Build history of the part. All positions in model axes, mm. A direction names the side the tool comes from. Give positions to 0.01 mm unless a question says otherwise; leave off trailing zeros. Order: outer loops, then holes, each group sorted by start corner. A loop starts at its lowest first (then second) coordinate and runs counter-clockwise, first axis right, second up. Notation, with made-up numbers: (29.5, 85) - (55.5, 85) arc R24 cw to (55.5, 107) - close; hole circle Ø4 at (-20, 47.5). An arc over 180 degrees is marked (long way). Answer in a Markdown table with one row per item.
```python
from build123d import *

# Parameters (mm, degrees)
EXTRUDE_1_DEPTH            = 25.5
CUT_EXTRUDE_1_DEPTH        = 23
CUT_EXTRUDE_START          = -1.5
CUT_EXTRUDE_2_DEPTH        = 1.5
SKETCH_3_W                 = 9
SKETCH_3_H                 = 1.25
EXTRUDE_2_DEPTH            = 7
SKETCH_4_W                 = 9
SKETCH_4_H                 = 3
EXTRUDE_3_DEPTH            = 1.25
CHAMFER_1_SIZE             = 1.3
CHAMFER_1_OF_MIRROR_1_SIZE = 1.3
MIRROR_START               = -31
MIRROR_4_DEPTH             = 9
MIRROR_START_2             = 22
MIRROR_4_2_DEPTH           = 9
SKETCH_5_W                 = 75
SKETCH_5_H                 = 50
CUT_EXTRUDE_3_DEPTH        = 0.5
CUT_EXTRUDE_4_DEPTH        = 115.248905903
CUT_EXTRUDE_4_DEPTH_BACK   = 0.5
SKETCH_6_W                 = 50
SKETCH_6_H                 = 14.5
CUT_EXTRUDE_5_REACH        = 98.222
SKETCH_7_R                 = 1.5
CUT_EXTRUDE_6_REACH        = 116.249
CUT_EXTRUDE_7_REACH        = 116.249


# Read off the part's stored shape, not the designer's step: Зеркальное отражение4
with BuildPart() as part:
    # Эскиз1 → Бобышка-Вытянуть1 (new body)
    with BuildSketch(Plane(origin=(0, 0, 0), x_dir=(1, 0, 0), z_dir=(0, 1, 0))):
        with BuildLine():
            Line((-43.5, 37.25), (43.5, 37.25))
            ThreePointArc((43.5, 37.25), (49.156854249, 34.906854249), (51.5, 29.25))
            Line((51.5, 29.25), (51.5, -29.25))
            ThreePointArc((51.5, -29.25), (49.156854249, -34.906854249), (43.5, -37.25))
            Line((43.5, -37.25), (-43.5, -37.25))
            ThreePointArc((-43.5, -37.25), (-49.156854249, -34.906854249), (-51.5, -29.25))
            Line((-51.5, -29.25), (-51.5, 29.25))
            ThreePointArc((-51.5, 29.25), (-49.156854249, 34.906854249), (-43.5, 37.25))
        make_face()
    extrude(amount=EXTRUDE_1_DEPTH)

    # Эскиз2 → Вырез-Вытянуть1 (cut)
    with BuildSketch(Plane(origin=(0, 25.5, 0), x_dir=(1, 0, 0), z_dir=(0, 1, 0))):
        with BuildLine():
            Line((-49, 29.25), (-49, -29.25))
            ThreePointArc((-49, -29.25), (-47.389087297, -33.139087297), (-43.5, -34.75))
            Line((-43.5, -34.75), (43.5, -34.75))
            ThreePointArc((43.5, -34.75), (47.389087297, -33.139087297), (49, -29.25))
            Line((49, -29.25), (49, 29.25))
            ThreePointArc((49, 29.25), (47.389087297, 33.139087297), (43.5, 34.75))
            Line((43.5, 34.75), (-43.5, 34.75))
            ThreePointArc((-43.5, 34.75), (-47.389087297, 33.139087297), (-49, 29.25))
        make_face()
    extrude(amount=-CUT_EXTRUDE_1_DEPTH, mode=Mode.SUBTRACT)

    # Эскиз2<3> → Вырез-Вытянуть2 (cut)
    with BuildSketch(Plane(origin=(0, 25.5, 0), x_dir=(1, 0, 0), z_dir=(0, 1, 0)).offset(CUT_EXTRUDE_START)):
        with BuildLine():
            Line((51.5, -29.25), (51.5, 29.25))
            ThreePointArc((51.5, 29.25), (49.156854249, 34.906854249), (43.5, 37.25))
            Line((43.5, 37.25), (-43.5, 37.25))
            ThreePointArc((-43.5, 37.25), (-49.156854249, 34.906854249), (-51.5, 29.25))
            Line((-51.5, 29.25), (-51.5, -29.25))
            ThreePointArc((-51.5, -29.25), (-49.156854249, -34.906854249), (-43.5, -37.25))
            Line((-43.5, -37.25), (43.5, -37.25))
            ThreePointArc((43.5, -37.25), (49.156854249, -34.906854249), (51.5, -29.25))
        make_face()
        with BuildLine():
            ThreePointArc((43.5, -36), (48.272970773, -34.022970773), (50.25, -29.25))
            Line((50.25, -29.25), (50.25, 29.25))
            ThreePointArc((50.25, 29.25), (48.272970773, 34.022970773), (43.5, 36))
            Line((43.5, 36), (-43.5, 36))
            ThreePointArc((-43.5, 36), (-48.272970773, 34.022970773), (-50.25, 29.25))
            Line((-50.25, 29.25), (-50.25, -29.25))
            ThreePointArc((-50.25, -29.25), (-48.272970773, -34.022970773), (-43.5, -36))
            Line((-43.5, -36), (43.5, -36))
        make_face(mode=Mode.SUBTRACT)
    extrude(amount=CUT_EXTRUDE_2_DEPTH, mode=Mode.SUBTRACT)

    # Эскиз3 → Бобышка-Вытянуть2 (add)
    with BuildSketch(Plane(origin=(0, 25.5, 0), x_dir=(1, 0, 0), z_dir=(0, 1, 0))):
        with Locations((-26.5, -35.375)):
            Rectangle(SKETCH_3_W, SKETCH_3_H)
    extrude_2 = extrude(amount=EXTRUDE_2_DEPTH)

    # Эскиз4 → Бобышка-Вытянуть3 (add, through all)
    with BuildSketch(Plane.XY.offset(36)):
        with Locations((-26.5, 31)):
            Rectangle(SKETCH_4_W, SKETCH_4_H)
    extrude_3 = extrude(amount=EXTRUDE_3_DEPTH)

    # Фаска1
    chamfer_1_edges = [part.edges().sort_by_distance(p)[0] for p in [
        (-26.5, 32.5, 37.25),
    ]]
    chamfer(chamfer_1_edges, length=CHAMFER_1_SIZE)

    # Зеркальное отражение1: Бобышка-Вытянуть2, Бобышка-Вытянуть3 across plane
    add(extrude_2.mirror(Plane(origin=(0, 0, 0), x_dir=(0, 0, 1), z_dir=(1, 0, 0))))
    add(extrude_3.mirror(Plane(origin=(0, 0, 0), x_dir=(0, 0, 1), z_dir=(1, 0, 0))))

    # Фаска1 of Зеркальное отражение1
    chamfer_1_of_mirror_1_edges = [part.edges().sort_by_distance(p)[0] for p in [
        (26.5, 32.5, 37.25),
    ]]
    chamfer(chamfer_1_of_mirror_1_edges, length=CHAMFER_1_OF_MIRROR_1_SIZE)

    # Зеркальное отражение4 outline → Зеркальное отражение4 (add)
    with BuildSketch(Plane.YZ.offset(MIRROR_START)):
        Polygon((25.5, -34.75), (25.5, -36), (29.5, -36), (29.5, -37.25), (31.2, -37.25), (32.5, -35.95), (32.5, -34.75), align=None)
    extrude(amount=MIRROR_4_DEPTH)

    # Mirror 4 2 outline → Mirror 4 2 (add)
    with BuildSketch(Plane.YZ.offset(MIRROR_START_2)):
        Polygon((25.5, -34.75), (25.5, -36), (29.5, -36), (29.5, -37.25), (31.2, -37.25), (32.5, -35.95), (32.5, -34.75), align=None)
    extrude(amount=MIRROR_4_2_DEPTH)

    # Эскиз5 → Вырез-Вытянуть3 (cut)
    with BuildSketch(Plane.XZ):
        Rectangle(SKETCH_5_W, SKETCH_5_H)
    extrude(amount=-CUT_EXTRUDE_3_DEPTH, mode=Mode.SUBTRACT)

    # Эскиз6 → Вырез-Вытянуть4 (cut, two sides: drawn at the far end of the back side and taken through both)
    with BuildSketch(Plane(origin=(51.5, 0, 0), x_dir=(0, 0, -1), z_dir=(1, 0, 0)).offset(-CUT_EXTRUDE_4_DEPTH_BACK)):
        with Locations((0, 16.75)):
            Rectangle(SKETCH_6_W, SKETCH_6_H)
    extrude(amount=CUT_EXTRUDE_4_DEPTH + CUT_EXTRUDE_4_DEPTH_BACK, mode=Mode.SUBTRACT)

    # Эскиз7 → Вырез-Вытянуть5 (cut, up to next)
    with BuildSketch(Plane(origin=(0, 0, -37.25), x_dir=(-1, 0, 0), z_dir=(0, 0, -1)), mode=Mode.PRIVATE) as cut_extrude_5_sk1:
        with Locations((15.3, 21.7)):
            Circle(SKETCH_7_R)
    cut_extrude_5_tool1 = extrude(cut_extrude_5_sk1.sketch, amount=-CUT_EXTRUDE_5_REACH, mode=Mode.PRIVATE) & part.part
    # Эскиз7 → Вырез-Вытянуть5 (cut, up to next)
    with BuildSketch(Plane(origin=(0, 0, -37.25), x_dir=(-1, 0, 0), z_dir=(0, 0, -1)), mode=Mode.PRIVATE) as cut_extrude_5_sk2:
        with Locations((7.3, 21.7)):
            Circle(SKETCH_7_R)
    cut_extrude_5_tool2 = extrude(cut_extrude_5_sk2.sketch, amount=-CUT_EXTRUDE_5_REACH, mode=Mode.PRIVATE) & part.part
    # Эскиз7 → Вырез-Вытянуть5 (cut, up to next)
    with BuildSketch(Plane(origin=(0, 0, -37.25), x_dir=(-1, 0, 0), z_dir=(0, 0, -1)), mode=Mode.PRIVATE) as cut_extrude_5_sk3:
        with Locations((-0.7, 21.7)):
            Circle(SKETCH_7_R)
    cut_extrude_5_tool3 = extrude(cut_extrude_5_sk3.sketch, amount=-CUT_EXTRUDE_5_REACH, mode=Mode.PRIVATE) & part.part
    # Эскиз7 → Вырез-Вытянуть5 (cut, up to next)
    with BuildSketch(Plane(origin=(0, 0, -37.25), x_dir=(-1, 0, 0), z_dir=(0, 0, -1)), mode=Mode.PRIVATE) as cut_extrude_5_sk4:
        with Locations((-8.7, 21.7)):
            Circle(SKETCH_7_R)
    cut_extrude_5_tool4 = extrude(cut_extrude_5_sk4.sketch, amount=-CUT_EXTRUDE_5_REACH, mode=Mode.PRIVATE) & part.part
    add(cut_extrude_5_tool1.solids().sort_by_distance((-15.3, 21.7, -37.25))[0], mode=Mode.SUBTRACT)
    add(cut_extrude_5_tool2.solids().sort_by_distance((-7.3, 21.7, -37.25))[0], mode=Mode.SUBTRACT)
    add(cut_extrude_5_tool3.solids().sort_by_distance((0.7, 21.7, -37.25))[0], mode=Mode.SUBTRACT)
    add(cut_extrude_5_tool4.solids().sort_by_distance((8.7, 21.7, -37.25))[0], mode=Mode.SUBTRACT)

    # Эскиз8 → Вырез-Вытянуть6 (cut, up to next)
    with BuildSketch(Plane.ZY.offset(51.5), mode=Mode.PRIVATE) as cut_extrude_6_sk1:
        with BuildLine():
            Line((-10.25, 16.5), (-22.25, 16.5))
            ThreePointArc((-22.25, 16.5), (-23.664213562, 17.085786438), (-24.25, 18.5))
            Line((-24.25, 18.5), (-24.25, 25.5))
            Line((-24.25, 25.5), (-8.25, 25.5))
            Line((-8.25, 25.5), (-8.25, 18.5))
            ThreePointArc((-8.25, 18.5), (-8.835786438, 17.085786438), (-10.25, 16.5))
        make_face()
    cut_extrude_6_tool1 = extrude(cut_extrude_6_sk1.sketch, amount=-CUT_EXTRUDE_6_REACH, mode=Mode.PRIVATE) & part.part
    # Эскиз8 → Вырез-Вытянуть6 (cut, up to next)
    with BuildSketch(Plane.ZY.offset(51.5), mode=Mode.PRIVATE) as cut_extrude_6_sk2:
        with BuildLine():
            Line((22.85, 16.5), (7.35, 16.5))
            ThreePointArc((7.35, 16.5), (5.935786438, 17.085786438), (5.35, 18.5))
            Line((5.35, 18.5), (5.35, 25.5))
            Line((5.35, 25.5), (24.85, 25.5))
            Line((24.85, 25.5), (24.85, 18.5))
            ThreePointArc((24.85, 18.5), (24.264213562, 17.085786438), (22.85, 16.5))
        make_face()
    cut_extrude_6_tool2 = extrude(cut_extrude_6_sk2.sketch, amount=-CUT_EXTRUDE_6_REACH, mode=Mode.PRIVATE) & part.part
    add(cut_extrude_6_tool1.solids().sort_by_distance((-51.5, 21.048907, -16.25))[0], mode=Mode.SUBTRACT)
    add(cut_extrude_6_tool2.solids().sort_by_distance((-51.5, 21.040042, 15.1))[0], mode=Mode.SUBTRACT)

    # Эскиз9 → Вырез-Вытянуть7 (cut, up to next)
    with BuildSketch(Plane(origin=(51.5, 0, 0), x_dir=(0, 0, -1), z_dir=(1, 0, 0)), mode=Mode.PRIVATE) as cut_extrude_7_sk1:
        with BuildLine():
            Line((-25.25, 25.5), (-9.25, 25.5))
            Line((-9.25, 25.5), (-9.25, 18.5))
            ThreePointArc((-9.25, 18.5), (-9.835786438, 17.085786438), (-11.25, 16.5))
            Line((-11.25, 16.5), (-23.25, 16.5))
            ThreePointArc((-23.25, 16.5), (-24.664213562, 17.085786438), (-25.25, 18.5))
            Line((-25.25, 18.5), (-25.25, 25.5))
        make_face()
    cut_extrude_7_tool1 = extrude(cut_extrude_7_sk1.sketch, amount=-CUT_EXTRUDE_7_REACH, mode=Mode.PRIVATE) & part.part
    # Эскиз9 → Вырез-Вытянуть7 (cut, up to next)
    with BuildSketch(Plane(origin=(51.5, 0, 0), x_dir=(0, 0, -1), z_dir=(1, 0, 0)), mode=Mode.PRIVATE) as cut_extrude_7_sk2:
        with BuildLine():
            Line((7.629289035, 25.5), (23.970741735, 25.5))
            Line((23.970741735, 25.5), (23.970741735, 18.5))
            ThreePointArc((23.970741735, 18.5), (23.384955297, 17.085786438), (21.970741735, 16.5))
            Line((21.970741735, 16.5), (9.629289035, 16.5))
            ThreePointArc((9.629289035, 16.5), (8.215075473, 17.085786438), (7.629289035, 18.5))
            Line((7.629289035, 18.5), (7.629289035, 25.5))
        make_face()
    cut_extrude_7_tool2 = extrude(cut_extrude_7_sk2.sketch, amount=-CUT_EXTRUDE_7_REACH, mode=Mode.PRIVATE) & part.part
    add(cut_extrude_7_tool1.solids().sort_by_distance((51.5, 21.048907, 17.25))[0], mode=Mode.SUBTRACT)
    add(cut_extrude_7_tool2.solids().sort_by_distance((51.5, 21.047873, -15.800015))[0], mode=Mode.SUBTRACT)


solid = part.part
```
1. Drop flat-ended pins along their axis: P1, Ø1.4, axis at x = -2.5, z = 35, coming from the +Y side; P2, Ø10, axis at x = 25, z = -11.5, coming from the -Y side; P3, Ø10.5, axis at x = 7, z = -28.5, coming from the +Y side. Give the stop position or say it passes through.
Check result:
| item | result |
|---|---|
| P1 | stops at y = 25.5 |
| P2 | stops at y = 0.5 |
| P3 | stops at y = 2.5 |
2. Which spindle directions (+Z, -Z, +X, -X, +Y, -Y) get a long thin tool onto all of the face, cutting with end or side? Do faces 1 (the face through (51, 15, 0)), 2 (the face through (44, 25.5, 35)), 3 (the face through (-43, 25.5, -35)), 4 (the face through (49, 12, 0)). Say none if no direction does.
Check result:
| item | result |
|---|---|
| face 1 | +X, +Y |
| face 2 | +Z, -Z, +X, +Y |
| face 3 | +Z, -Z, -X, +Y |
| face 4 | +Y |
3. Cut at B-B on x = 0.7. Write the cut outline in (y, z), and give its area (3 significant figures).
Check result:
| item | result |
|---|---|
| outline | (0, -37.25) - (20.2, -37.25) - (20.2, -34.75) - (2.5, -34.75) - (2.5, 34.75) - (25.5, 34.75) - (25.5, 36) - (24, 36) - (24, 37.25) - (0, 37.25) - (0, 25) - (0.5, 25) - (0.5, -25) - (0, -25) - close; (23.2, -37.25) - (24, -37.25) - (24, -36) - (25.5, -36) - (25.5, -34.75) - (23.2, -34.75) - close |
| area | 265 mm² |
4. Probe line 1 (X direction, y = 15.5, z = -18.5); line 2 (X direction, y = 5.5, z = -14.5); line 3 (Z direction, x = 12, y = 16.5). List the from-to ranges inside material, lowest first.
Check result:
| item | result |
|---|---|
| line 1 | x = -51.5 to -49, 49 to 51 |
| line 2 | x = -51.5 to -49, 49 to 51.5 |
| line 3 | z = -37.25 to -34.75, 34.75 to 37.25 |
5. Cut at D-D on y = 21.7. Count the separate pieces of the cut face and the enclosed holes in it, and give its area (3 significant figures).
Check result:
| item | result |
|---|---|
| separate pieces | 8 |
| enclosed holes | 0 |
| area | 625 mm² |
6. Cut at C-C on x = -29. Write the cut outline in (y, z).
Check result:
| item | result |
|---|---|
| outline | (0, -37.25) - (24, -37.25) - (24, -36) - (29.5, -36) - (29.5, -37.25) - (31.2, -37.25) - (32.5, -35.95) - (32.5, -34.75) - (2.5, -34.75) - (2.5, 34.75) - (32.5, 34.75) - (32.5, 35.95) - (31.2, 37.25) - (29.5, 37.25) - (29.5, 36) - (24, 36) - (24, 37.25) - (0, 37.25) - (0, 25) - (0.5, 25) - (0.5, -25) - (0, -25) - close |
7. Cut at A-A on y = 28. Write the cut outline in (x, z), and give its area (3 significant figures).
Check result:
| item | result |
|---|---|
| outline | (-31, -36) - (-22, -36) - (-22, -34.75) - (-31, -34.75) - close; (-31, 34.75) - (-22, 34.75) - (-22, 36) - (-31, 36) - close; (22, -36) - (31, -36) - (31, -34.75) - (22, -34.75) - close; (22, 34.75) - (31, 34.75) - (31, 36) - (22, 36) - close |
| area | 45.0 mm² |
8. Two-plate mould, pull along X, no slides. Class faces 5 (the face through (49.219, 11.832, 34.844)), 6 (the face through (47.43, 14.16, -33.1)), 7 (the face through (-50, 22, 24.85)): +X half, -X half, draft (parallel to the pull), parting line (faces both ways), or undercut.
Check result:
| item | result |
|---|---|
| face 5 | +X half |
| face 6 | undercut |
| face 7 | draft |
